The figure shows three views and two pictorial views of one solid part (mm, origin at its lowest corner). Answer the questions. Coordinates: 2 decimals unless noted, no trailing zeros. Write each loop counter-clockwise with the first axis right and the second up, starting at its lowest first coordinate (ties: lowest second). Pieces come first, ordered by that corner, then holes.
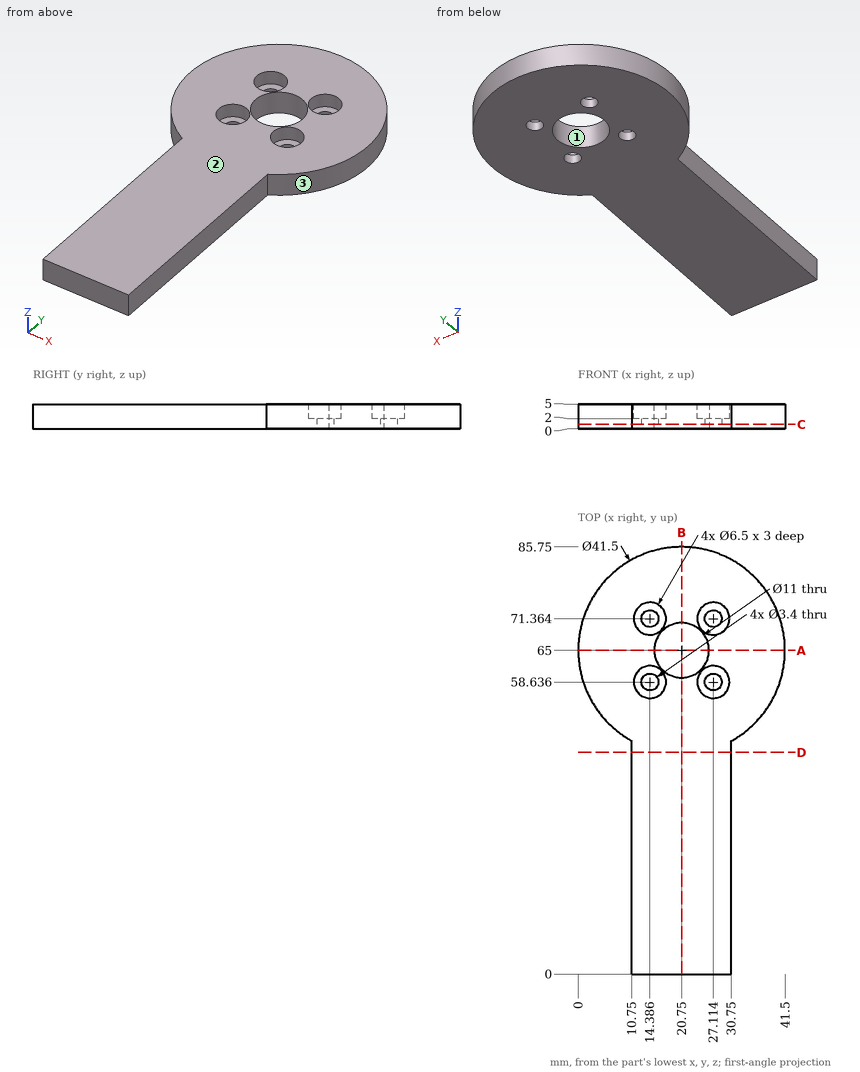
1. Section D-D on y = 44.5 is taken. Give the vertices of the cut face in (x, z).
Results found:
outline: (10.75, 0) - (30.75, 0) - (30.75, 5) - (10.75, 5) - close
2. For a pull along X with two mould halves and no side action, classify the marked faces 1, 2 and 3 as pulls with the +X half, pulls with the -X half, needs draft (parallel to the pull), parting line crosses it, or undercut.
Results found:
face 1: undercut
face 2: needs draft
face 3: parting line crosses it
3. Section C-C on z = 0.9 is taken. Give the vertices of the cut face in (x, y).
Results found:
outline: (10.75, 0) - (30.75, 0) - (30.75, 46.82) arc R20.75 ccw (long way) to (10.75, 46.82) - close; hole circle Ø3.4 at (14.39, 58.64); hole circle Ø3.4 at (14.39, 71.36); hole circle Ø11 at (20.75, 65); hole circle Ø3.4 at (27.11, 58.64); hole circle Ø3.4 at (27.11, 71.36)
4. Section B-B on x = 20.75 is taken. Give the vertices of the cut face in (y, z).
Results found:
outline: (0, 0) - (59.5, 0) - (59.5, 5) - (0, 5) - close; (70.5, 0) - (85.75, 0) - (85.75, 5) - (70.5, 5) - close
5. Section A-A on y = 65 is taken. Give the vertices of the cut face in (x, z).
Results found:
outline: (0, 0) - (15.25, 0) - (15.25, 5) - (0, 5) - close; (26.25, 0) - (41.5, 0) - (41.5, 5) - (26.25, 5) - close
6. Flat-ended cylindrical pins translate along their axes: P1, Ø2.5, axis at y = 19, z = 1.5, coming from the +X side; P2, Ø1.5, axis at y = 68.5, z = 4, coming from the +X side; P3, Ø1.5, axis at x = 34.5, z = 2, coming from the +Y side; P4, Ø3, axis at x = 14.39, y = 71.36, coming from the +Z side. Find the tip coordinate at first contact, or state that the pin passes through.
Results found:
P1: stops at x = 30.75
P2: stops at x = 41.32
P3: stops at y = 81.17
P4: passes through
7. Find the intervals of material crossed by L1, parallel to Y at x = 26.5, z = 1.35; L2, parallel to Y at x = 29, z = 2.65; L3, parallel to Y at x = 16.5, z = 2.75, in increasing order.
Results found:
L1: y = 0 to 57.05, 60.22 to 69.78, 72.95 to 84.94
L2: y = 0 to 55.99, 61.28 to 68.72, 74.01 to 84.04
L3: y = 0 to 56.17, 61.1 to 61.51, 68.49 to 68.9, 73.83 to 85.31
